```python
from build123d import *

# Parameters (mm, degrees)
F0_W      = 95
F0_H      = 100
F1_DEPTH  = 5
F3_DEPTH  = 5
F5_DEPTH  = 5
F7_DEPTH  = 5
F8_R      = 10
F10_DEPTH = 10
F12_DEPTH = 10


with BuildPart() as f1:
    # F0 (on Top) → F1 (new body)
    with BuildSketch(Plane.XY):
        with Locations((47.5, 50)):
            Rectangle(F0_W, F0_H)
    extrude(amount=F1_DEPTH)

    # F2 (on face) → F3 (join)
    with BuildSketch(Plane(origin=(0, 0, 0), x_dir=(0, -1, 0), z_dir=(-1, 0, 0))):
        with BuildLine():
            Line((0, 5), (0, 35.901699))
            ThreePointArc((0, 35.901699), (-25.589962, 50.916501), (-55, 54.833148))
            Line((-55, 54.833148), (-55, 80))
            Line((-55, 80), (-85, 80))
            Line((-85, 80), (-85, 46.332496))
            ThreePointArc((-85, 46.332496), (-92.818809, 41.57556), (-100, 35.901699))
            Line((-100, 35.901699), (-100, 5))
            Line((-100, 5), (0, 5))
        make_face()
    extrude(amount=-F3_DEPTH)

    # F4 (on face) → F5 (join)
    with BuildSketch(Plane.XZ):
        Polygon((5, 70), (5, 5), (95, 5), (95, 70), (80, 70), (80, 20), (40, 20), (40, 70), align=None)
    extrude(amount=-F5_DEPTH)

    # F6 (on face) → F7 (join)
    with BuildSketch(Plane(origin=(0, 100, 0), x_dir=(-1, 0, 0), z_dir=(0, 1, 0))):
        Polygon((-95, 5), (-5, 5), (-5, 70), (-20, 70), (-20, 20), (-60, 20), (-60, 70), (-95, 70), align=None)
    extrude(amount=-F7_DEPTH)

    # F8
    f8_edges = [f1.edges().sort_by_distance(p)[0] for p in [
        (20, 97.5, 20),
        (40, 2.5, 20),
        (60, 97.5, 20),
        (80, 2.5, 20),
    ]]
    fillet(f8_edges, radius=F8_R)

    # F9 (on face) → F10 (join)
    with BuildSketch(Plane.XY.offset(5)):
        Polygon((10, 85), (10, 50), (30, 50), (30, 75), (60, 75), (60, 85), align=None)
    extrude(amount=F10_DEPTH)

    # F11 (on face) → F12 (cut)
    with BuildSketch(Plane.XY.offset(15)):
        Polygon((57.999999, 82.999999), (12.000001, 82.999999), (12.000001, 52.000001), (27.999999, 52.000001), (27.999999, 77.000001), (57.999999, 77.000001), align=None)
    extrude(amount=-F12_DEPTH, mode=Mode.SUBTRACT)


solid = f1.part
```
Can you work these out from the model? Positions are in its coordinate system, mm. A direction names the side the tool comes from. Give positions to 0.01 mm unless a question says otherwise; leave off trailing zeros. Order: outer loops, then holes, each group sorted by start corner. A loop starts at its lowest first (then second) coordinate and runs counter-clockwise, first axis right, second up. Notation, with made-up numbers: M -15,21.25 L -7,21.25 A25 cw -7,40.25 Z; hole C 84.25,9 d3. An arc over 180 degrees is marked long. Write item = value, one per line. Start each with the question number.
Q1. Suppose I cut it at C-C (y = 62). Write out the boundary of the cut face in (x, z).
Q2. Suppose I cut it at B-B (x = 37). Write out the boundary of the cut face in (y, z), plus the area to 3 significant figures.
Q3. I need wall thicknesses on probe 1 along Y at (x, z) = (82, 57.5); probe 2 along Z at (x, y) = (45.5, 18.5); probe 3 along Y at (x, z) = (72.5, 37). Which ranges of each line are inside material? Lowest first, please. Write a range as [from, to].
Q4. Will these pins go through, and if not, where does the flat tip stop? pin 1 Ø3 at (y, z) = (17, 22.5) entering from +X; pin 2 Ø1.5 at (x, z) = (36, 58) entering from -Y; pin 3 Ø1 at (x, z) = (77.5, 65.5) entering from -Y; pin 4 Ø2.5 at (y, z) = (2.5, 43) entering from -X.
Q5. Suppose I cut it at A-A (z = 33). Write out the boundary of the cut face in (x, y), plus the area to 3 significant figures.
Q6. We'd pull the mould along Y, two halves only. Please class faces 5 (the cylindrical face through (2.46, 92.71, 41.65)), 6 (the flat face through (36, 0, 28)), 7 (the flat face through (61, 95, 31)): pulls with the +Y half, pulls with the -Y half, needs draft (parallel to the pull), parting line crosses it, or undercut.
Q7. For faces 1 (the cylindrical face through (57.15, 97.46, 23.01)), 2 (the flat face through (31.2, 75.4, 15)), 3 (the flat face through (12, 68, 10)), 4 (the cylindrical face through (23.01, 97.46, 22.85)), which set-ups out of +Z, -Z, +X, -X, +Y, -Y let a thin tool reach every point of the face, with its end or its side?
Q8. Suppose I cut it at D-D (z = 65.5). Write out the boundary of the cut face in (x, y), plus the area to 3 significant figures.
Check result:
q1.outline = M 0,0 L 95,0 L 95,5 L 30,5 L 30,15 L 28,15 L 28,5 L 12,5 L 12,15 L 10,15 L 10,5 L 5,5 L 5,80 L 0,80 Z
q2.outline = M 0,0 L 100,0 L 100,20 L 95,20 L 95,5 L 85,5 L 85,15 L 83,15 L 83,5 L 77,5 L 77,15 L 75,15 L 75,5 L 5,5 L 5,70 L 0,70 Z
q2.area = 940 mm2
q3.probe_1 = [0, 5], [95, 100]
q3.probe_2 = [0, 5]
q3.probe_3 = [95, 100]
q4.pin_1 = 5
q4.pin_2 = 0
q4.pin_3 = 95
q4.pin_4 = 5
q5.outline = M 0,0 L 40,0 L 40,5 L 5,5 L 5,95 L 20,95 L 20,100 L 0,100 Z; M 60,95 L 95,95 L 95,100 L 60,100 Z; M 80,0 L 95,0 L 95,5 L 80,5 Z
q5.area = 1,000 mm2
q6.face_5 = pulls with the +Y half
q6.face_6 = pulls with the -Y half
q6.face_7 = undercut
q7.face_1 = +Z, +Y, -Y
q7.face_2 = +Z, +X
q7.face_3 = +Z
q7.face_4 = +Z, +Y
q8.outline = M 0,55 L 5,55 L 5,85 L 0,85 Z; M 5,0 L 40,0 L 40,5 L 5,5 Z; M 5,95 L 20,95 L 20,100 L 5,100 Z; M 60,95 L 95,95 L 95,100 L 60,100 Z; M 80,0 L 95,0 L 95,5 L 80,5 Z
q8.area = 650 mm2
